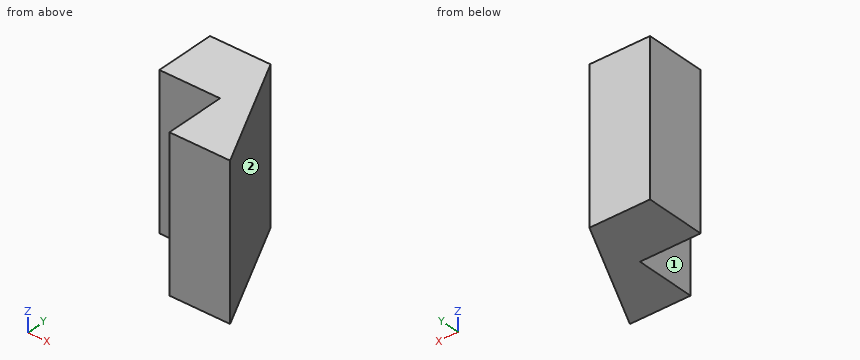
from build123d import *

# Parameters (mm, degrees)
BOSS_EXTRUDE1_DEPTH = 25


with BuildPart() as part:
    # Sketch1 → Boss-Extrude1 (new body)
    with BuildSketch(Plane.XY):
        Polygon((-10, 20), (0, 20), (10, 0), (0, 0), (0, 10), (-10, 10), align=None)
    extrude(amount=BOSS_EXTRUDE1_DEPTH)


solid = part.part
Read the model definition and answer for the solid it produces. Units are mm, in the model's axes. Face numbers are marked on the shaded views. A direction names the side the tool comes from. Give positions to 0.01 mm unless a question says otherwise; leave off trailing zeros. Write each loop counter-clockwise with the first axis right and the second up, starting at its lowest first coordinate (ties: lowest second). Pieces come first, ordered by that corner, then holes. Notation, with made-up numbers: (33.5, 6.5) - (87.5, 6.5) arc R32 cw to (87.5, 40.5) - close; hole circle Ø5 at (11, 30). An arc over 180 degrees is marked (long way). Use CSV: the item, a comma, the result in double quotes. Start each with the question number.
(1) Consider line 1 along Y through (x, z) = (-4.25, 21.5); line 2 along X through (y, z) = (3.75, 13.75) (3 decimals); line 3 along X through (y, z) = (2, 15.75). Determine where each line is inside the solid, lowest interval first.
(2) Find section B-B (y = 18). Give the vertices of the cut face in (x, z), plus the area to 3 significant figures.
(3) For the marked faces 1 and 2, determine the directions among +Z, -Z, +X, -X, +Y, -Y from which every point of the face is accessible in a straight line to the end or side of a thin tool.
(4) Given P1, Ø12, axis at x = 6.5, z = 5, coming from the +Y side; P2, Ø2, axis at x = -7, z = 7, coming from the -Y side; P3, Ø11, axis at y = 5.5, z = 7, coming from the -X side; P4, Ø8, axis at y = 8, z = 2.5, coming from the +X side, each flat-ended and moving along its own axis, determine where each tip first touches the part or whether it passes through.
(5) Find section C-C (x = 4.5). Give the vertices of the cut face in (y, z), plus the area to 3 significant figures.
(6) Find section A-A (z = 1.5). Give the vertices of the cut face in (x, y).
Findings below:
1,line 1,"10 to 20"
1,line 2,"0 to 8.125"
1,line 3,"0 to 9"
2,outline,"(-10, 0) - (1, 0) - (1, 25) - (-10, 25) - close"
2,area,"275 mm2"
3,face 1,"+Z, -Z, -X, -Y"
3,face 2,"+Z, -Z, +X, +Y"
4,P1,"y = 19"
4,P2,"y = 10"
4,P3,"x = -10"
4,P4,"x = 8"
5,outline,"(0, 0) - (11, 0) - (11, 25) - (0, 25) - close"
5,area,"275 mm2"
6,outline,"(-10, 10) - (0, 10) - (0, 0) - (10, 0) - (0, 20) - (-10, 20) - close"
